Part model, mm, in its own coordinate system. A direction names the side the tool comes from. Round coordinates to 2 decimals unless told otherwise and drop trailing zeros. Write each loop counter-clockwise with the first axis right and the second up, starting at its lowest first coordinate (ties: lowest second). Pieces come first, ordered by that corner, then holes.
1) Drill centre lines: L1, parallel to Z at x = 46, y = 4; L2, parallel to Y at x = -7.5, z = 22; L3, parallel to X at y = 23.75, z = 10.5. Where is each one in solid material? Low to high.
2) Pull direction Y, two halves, no side cores. Call faces 1 (the flat face through (92, 13, 7)), 2 (the cylindrical face through (95.854, 5.16, 21.246)), 3 (the flat face through (9, 18, 11)): +Y half, -Y half, draft (parallel to the pull), parting line (faces both ways), or undercut.
3) Saw through at C-C on z = 13.75. Write the cut outline in (x, y).
4) Saw through at D-D on y = 10.5. Write the cut outline in (x, z).
5) Which spindle directions (+Z, -Z, +X, -X, +Y, -Y) get a long thin tool onto all of the face, cutting with end or side? Do faces 4 (the flat face through (0, 14, 7)), 5 (the flat face through (100, 14, 15)), 6 (the cylindrical face through (97.724, 18.811, 19.569)), 7 (the cylindrical face through (5.24, 18.35, 7.61)). Say none if no direction does.
6) Saw through at A-A on y = 5. Write the cut outline in (x, z).
7) Saw through at B-B on x = 46. Write the cut outline in (y, z).
8) Flat gauge pins, fed straight in: pin 1 (5 mm diameter, centred on x = 12, z = 18.5, fed in from +Y); pin 2 (7.5 mm diameter, centred on x = -10, y = 13.5, fed in from -Z); pin 3 (1.7 mm diameter, centred on y = 21.5, z = 6, fed in from -X); pin 4 (5 mm diameter, centred on x = 86.5, z = 5.5, fed in from -Y). Where does each tip first touch, or does it go through?
Autodesk Inventor part; units mm, degrees
ref_plane "Work Plane1" through (77, 0, 15) normal (1, 0, 0) x (0, 0, -1)
ref_plane "Work Plane2" through (15, 0, 0) normal (-1, 0, 0) x (0, 0, 1)
ref_plane "YZ Plane" through (0, 0, 0) normal (1, 0, 0) x (0, 1, 0)
sketch "Sketch1" plane through (0, 0, 0) normal (0, 0, 1) x (1, 0, 0)
  line L0 (0, 0) -> (92, 0)
  line L1 (92, 0) -> (92, 12)
  line L2 (92, 12) -> (0, 12)
  line L3 (0, 12) -> (0, 0)
  dimension "d0" = 92
  dimension "d1" = 12
extrude "Extrusion1" add sketch "Sketch1" along normal blind 30
sketch "Sketch3" plane through (0, 12, 30) normal (0, 1, 0) x (1, 0, 0)
  line L0 (0, 30) -> (0, 0)
  line L1 (92, 30) -> (0, 30)
  circle A0 centre (46, 14.15) radius 7.9
  point P0 (0, 17)
  point P1 (107, 32)
  point P2 (15, 32)
  dimension "d8" = 15.8
  dimension "d9" = 15.85
  dimension "d10" = 46
extrude "Extrusion3" cut sketch "Sketch3" against normal up to next
sketch "Sketch4" plane through (0, 12, 0) normal (0, 1, 0) x (1, 0, 0)
  line L0 (0, 0) -> (0, -30)
  line L1 (92, 0) -> (92, -30)
  line L2 (0, -30) -> (-15, -15)
  line L3 (-15, -15) -> (0, -15)
  line L4 (92, -30) -> (107, -15)
  line L5 (107, -15) -> (92, -15)
  dimension "d13" = 45
  dimension "d14" = 45
extrude "Extrusion4" add sketch "Sketch4" against normal up to surface (12 mm away)
sketch "Sketch5" plane through (0, 0, 0) normal (1, 0, 0) x (0, 1, 0)
  line L0 (0, 15) -> (0, 30)
  line L1 (12, 30) -> (0, 30)
  line L2 (12, 15) -> (12, 30)
  line L3 (12, 15) -> (0, 15)
  line L4 (12, 15) -> (27, 15)
  line L5 (27, 15) -> (12, 30)
  point P0 (0, 0)
  dimension "d17" = 15
extrude "Extrusion5" add sketch "Sketch5" against normal up to surface contours L2 L5 L4 surface through (0, 12, 30) normal (-0.7071, 0, 0.7071)
sketch "Sketch6" plane through (92, 0, 0) normal (1, 0, 0) x (0, 0, -1)
  line L0 (-30, 0) -> (-15, 0)
  line L1 (-15, 12) -> (-15, 0)
  line L2 (-30, 12) -> (-15, 12)
  line L3 (-30, 0) -> (-30, 12)
  line L4 (-15, 12) -> (-15, 27)
  line L5 (-15, 27) -> (-30, 12)
  dimension "d20" = 15
extrude "Extrusion6" add sketch "Sketch6" along normal up to surface contours L5 L4 L2 surface through (107, 12, 15) normal (0.7071, 0, 0.7071)
sketch "Sketch7" plane through (0, 0, 0) normal (0, 0, -1) x (-1, 0, 0)
  line L0 (-92, 12) -> (0, 12)
  line L1 (-92, 12) -> (-92, 27)
  line L2 (-92, 27) -> (-77, 12)
  line L3 (0, 12) -> (0, 27)
  line L4 (0, 27) -> (-15, 12)
  dimension "d23" = 15
  dimension "d24" = 15
extrude "Extrusion7" add sketch "Sketch7" against normal up to surface surface through (92, 27, 15) normal (0, 0.7071, 0.7071)
sketch "Sketch8" plane through (0, 0, 30) normal (0, 0, 1) x (1, 0, 0)
  line L0 (-15, 0) -> (0, 0)
  line L1 (0, 12) -> (0, 0)
  line L2 (-15, 27) -> (0, 12)
  line L3 (-15, 0) -> (-15, 27)
  line L4 (92, 0) -> (107, 0)
  line L5 (107, 27) -> (107, 0)
  line L6 (92, 12) -> (107, 27)
  line L7 (92, 0) -> (92, 12)
  circle A0 centre (-7.5, 5) radius 1.75
  circle A1 centre (-7.5, 22) radius 1.75
  circle A2 centre (99.5, 22) radius 1.75
  circle A3 centre (99.5, 5) radius 1.75
  line L8 (92, 27) -> (107, 27)
  dimension "d27" = 3.5
  dimension "d28" = 7.5
  dimension "d29" = 7.5
  dimension "d30" = 5
  dimension "d31" = 5
extrude "Extrusion8" cut sketch "Sketch8" against normal up to surface (15 mm away) contours A0 | A1 | A2 | A3
sketch "Sketch9" plane through (0, 0, 30) normal (0, 0, 1) x (1, 0, 0)
  circle A0 centre (-7.5, 22) radius 1.75
  circle A1 centre (-7.5, 5) radius 1.75
  circle A2 centre (99.5, 22) radius 1.75
  circle A3 centre (99.5, 5) radius 1.75
  circle A4 centre (-7.5, 22) radius 3.65
  circle A5 centre (-7.5, 5) radius 3.65
  circle A6 centre (99.5, 22) radius 3.65
  circle A7 centre (99.5, 5) radius 3.65
  dimension "d34" = 7.3
extrude "Extrusion9" cut sketch "Sketch9" against normal blind 12
ref_plane "Work Plane1" through (77, 0, 15) normal (1, 0, 0) x (0, 0, -1)
sketch "Sketch10" plane through (77, 0, 15) normal (1, 0, 0) x (0, 0, -1)
  line L0 (-15, 12) -> (0, 27)
  line L1 (15, 27) -> (0, 27)
  line L2 (15, 12) -> (15, 27)
  line L3 (-15, 12) -> (15, 12)
  circle A0 centre (7.5, 22) radius 1.75
  circle A1 centre (7.5, 22) radius 3.65
  point P0 (15, 0)
  dimension "d38" = 3.5
  dimension "d39" = 7.3
  dimension "d40" = 5
  dimension "d41" = 7.5
extrude "Extrusion10" cut sketch "Sketch10" along normal up to surface (15 mm away) contours A0
sketch "Sketch11" plane through (77, 0, 15) normal (1, 0, 0) x (0, 0, -1)
  circle A0 centre (7.5, 22) radius 1.75
  circle A1 centre (7.5, 22) radius 3.65
  point P0 (15, 0)
  dimension "d44" = 7.3
extrude "Extrusion11" cut sketch "Sketch11" along normal blind 12
ref_plane "Work Plane2" through (15, 0, 0) normal (-1, 0, 0) x (0, 0, 1)
sketch "Sketch12" plane through (15, 0, 0) normal (-1, 0, 0) x (0, 0, 1)
  line L0 (15, 27) -> (30, 12)
  line L1 (0, 12) -> (30, 12)
  line L2 (0, 27) -> (0, 12)
  line L3 (0, 27) -> (15, 27)
  circle A0 centre (7.5, 22) radius 1.75
  point P0 (0, 0)
  dimension "d48" = 3.5
  dimension "d49" = 7.5
  dimension "d50" = 5
extrude "Extrusion12" cut sketch "Sketch12" along normal up to surface (15 mm away) contours A0
sketch "Sketch13" plane through (15, 0, 0) normal (-1, 0, 0) x (0, 0, 1)
  circle A0 centre (7.5, 22) radius 1.75
  circle A1 centre (7.5, 22) radius 1.75
  circle A2 centre (7.5, 22) radius 3.65
  point P0 (0, 0)
  dimension "d53" = 7.3
extrude "Extrusion13" cut sketch "Sketch13" along normal blind 12
properties part number "ZAxisNutMount"
Completed:
1. L1: z = 0 to 7.95, 23.75 to 30
1. L2: y = 0 to 1.35, 8.65 to 18.35
1. L3: x = 0 to 3, 89 to 92
2. face 1: draft
2. face 2: undercut
2. face 3: +Y half
3. outline: (0, 0) - (38.38, 0) - (38.38, 12) - (15, 12) - (0, 27) - close; (53.62, 0) - (92, 0) - (92, 27) - (77, 12) - (53.62, 12) - close
4. outline: (-15, 15) - (0, 15) - (0, 0) - (92, 0) - (92, 15) - (107, 15) - (92, 30) - (0, 30) - close; hole circle Ø15.8 at (46, 15.85)
5. face 4: -Z, -X, +Y, -Y
5. face 5: -Z, +X, +Y, -Y
5. face 6: +Z
5. face 7: none
6. outline: (-15, 15) - (-9.25, 15) - (-9.25, 18) - (-11.15, 18) - (-11.15, 18.85) - close; (-5.75, 15) - (0, 15) - (0, 0) - (92, 0) - (92, 15) - (97.75, 15) - (97.75, 18) - (95.85, 18) - (95.85, 26.15) - (92, 30) - (0, 30) - (-3.85, 26.15) - (-3.85, 18) - (-5.75, 18) - close; (101.25, 15) - (107, 15) - (103.15, 18.85) - (103.15, 18) - (101.25, 18) - close; hole circle Ø15.8 at (46, 15.85)
7. outline: (0, 0) - (12, 0) - (12, 7.95) - (0, 7.95) - close; (0, 23.75) - (12, 23.75) - (12, 30) - (0, 30) - close
8. pin 1: stops at y = 17.5
8. pin 2: stops at z = 15
8. pin 3: stops at x = 0
8. pin 4: stops at y = 0
